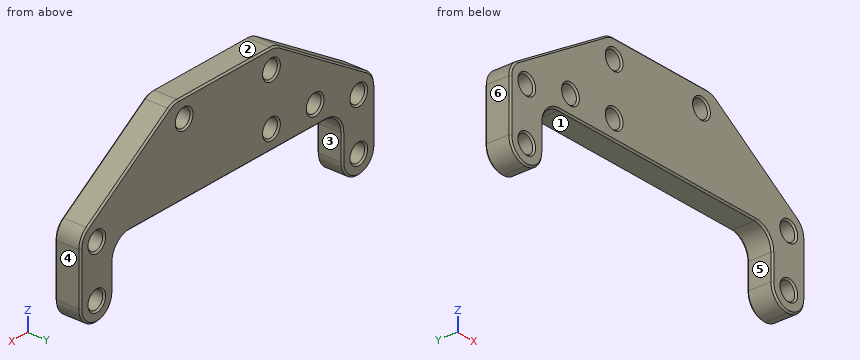
```python
from build123d import *

# Parameters (mm, degrees)
SKETCH1_R           = 2.1828125
BOSS_EXTRUDE1_DEPTH = 3.175
FILLET1_R           = 4.7625
CHAMFER1_SIZE       = 0.396875


with BuildPart() as part:
    # Sketch1 → Boss-Extrude1 (new, symmetric)
    with BuildSketch(Plane(origin=(0, 0, 0), x_dir=(1, 0, 0), z_dir=(0, 1, 0))):
        Polygon((-33.3375, 7.9375), (-33.3375, 23.8125), (-42.8625, 23.8125), (-42.8625, 3.710395607), (-14.065867028, -14.2875), (15.876245853, -14.2875), (42.8625, 3.710395607), (42.8625, 23.8125), (33.3375, 23.8125), (33.3375, 7.9375), align=None)
        with Locations(Location((-38.1, 6.35, 0), (0, 0, 270))):
            Circle(SKETCH1_R, mode=Mode.SUBTRACT)
        with Locations(Location((-38.1, 19.05, 0), (0, 0, 270))):
            Circle(SKETCH1_R, mode=Mode.SUBTRACT)
        with Locations(Location((38.1, 19.05, 0), (0, 0, 270))):
            Circle(SKETCH1_R, mode=Mode.SUBTRACT)
        with Locations(Location((38.1, 6.35, 0), (0, 0, 270))):
            Circle(SKETCH1_R, mode=Mode.SUBTRACT)
        with Locations(Location((-25.4, 3.175, 0), (0, 0, 270))):
            Circle(SKETCH1_R, mode=Mode.SUBTRACT)
        with Locations(Location((-12.7, 3.175, 0), (0, 0, 270))):
            Circle(SKETCH1_R, mode=Mode.SUBTRACT)
        with Locations(Location((-12.7, -9.525, 0), (0, 0, 270))):
            Circle(SKETCH1_R, mode=Mode.SUBTRACT)
        with Locations(Location((12.7, -9.525, 0), (0, 0, 270))):
            Circle(SKETCH1_R, mode=Mode.SUBTRACT)
    extrude(amount=BOSS_EXTRUDE1_DEPTH, both=True)

    # Fillet1
    fillet1_edges = [part.edges().sort_by_distance(p)[0] for p in [
        (42.8625, 0, -3.710395607),
        (15.876245853, 0, 14.2875),
        (-14.065867028, 0, 14.2875),
        (-42.8625, 0, -3.710395607),
        (-33.3375, 0, -23.8125),
        (-42.8625, 0, -23.8125),
        (42.8625, 0, -23.8125),
        (33.3375, 0, -23.8125),
        (33.3375, 0, -7.9375),
        (-33.3375, 0, -7.9375),
    ]]
    fillet(fillet1_edges, radius=FILLET1_R - 0.0001)  # a hair under: the kernel refuses the full size

    # Chamfer1
    chamfer1_edges = [part.edges().sort_by_distance(p)[0] for p in [
        (-38.1, -3.175, -8.5328125),
        (-38.1, 3.175, -8.5328125),
        (-38.1, -3.175, -21.2328125),
        (-38.1, 3.175, -21.2328125),
        (38.1, -3.175, -21.2328125),
        (38.1, 3.175, -21.2328125),
        (38.1, -3.175, -8.5328125),
        (38.1, 3.175, -8.5328125),
        (-12.7, -3.175, -5.3578125),
        (-12.7, 3.175, -5.3578125),
        (-25.4, -3.175, -5.3578125),
        (-25.4, 3.175, -5.3578125),
        (12.7, -3.175, 7.3421875),
        (12.7, 3.175, 7.3421875),
        (-12.7, -3.175, 7.3421875),
        (-12.7, 3.175, 7.3421875),
        (42.8625, -3.175, -12.654350033),
        (42.8625, 3.175, -12.654350033),
        (28.909389934, -3.175, 5.595327855),
        (0.866903869, -3.175, 14.2875),
        (-27.924131292, -3.175, 5.626084835),
        (-42.8625, -3.175, -12.700022288),
        (-33.3375, -3.175, -15.875),
        (0, -3.175, -7.9375),
        (33.3375, -3.175, -15.875),
        (34.732374665, -3.175, -22.417625335),
        (41.467625335, -3.175, -22.417625335),
        (-41.467625335, -3.175, -22.417625335),
        (-34.732374665, -3.175, -22.417625335),
        (-42.265497353, -3.175, -4.041282917),
        (-14.01293908, -3.175, 14.102951029),
        (15.814317137, -3.175, 14.083030095),
        (42.299190555, -3.175, -4.011804065),
        (28.909389934, 3.175, 5.595327855),
        (33.3375, 3.175, -15.875),
        (0, 3.175, -7.9375),
        (-33.3375, 3.175, -15.875),
        (-42.8625, 3.175, -12.700022288),
        (-27.924131292, 3.175, 5.626084835),
        (0.866903869, 3.175, 14.2875),
        (34.732374665, 3.175, -22.417625335),
        (41.467625335, 3.175, -22.417625335),
        (-41.467625335, 3.175, -22.417625335),
        (-34.732374665, 3.175, -22.417625335),
        (-42.265497353, 3.175, -4.041282917),
        (-14.01293908, 3.175, 14.102951029),
        (15.814317137, 3.175, 14.083030095),
        (42.299190555, 3.175, -4.011804065),
        (31.942625335, -3.175, -9.332374665),
        (31.942625335, 3.175, -9.332374665),
        (-31.942625335, -3.175, -9.332374665),
        (-31.942625335, 3.175, -9.332374665),
    ]]
    chamfer(chamfer1_edges, length=CHAMFER1_SIZE)


solid = part.part
```
Check sheet for the modelled part. Datum: model origin and axes. Units: mm. Face numbers are marked on the shaded views. A direction names the side the tool comes from. Coordinates: 2 decimals unless noted, no trailing zeros. Order: outer loops, then holes, each group sorted by start corner. A loop starts at its lowest first (then second) coordinate and runs counter-clockwise, first axis right, second up. Notation, with made-up numbers: M 79,-12.5 L 126,-12.5 A16 ccw 126,-0.5 Z; hole C -19.5,-6 d7. An arc over 180 degrees is marked long. One line per question, with ' | ' between items. Start each with the question number.
Item 1: Gauge pin test, flat ends, axial feed: P1, Ø4, axis at x = 38.1, z = -19.05, coming from the +Y side; P2, Ø2, axis at y = -1.5, z = -0.5, coming from the +X side; P3, Ø2, axis at x = 19, y = -2, coming from the +Z side; P4, Ø5, axis at x = -38.1, z = -6.35, coming from the +Y side. Record the tip position at first contact, or that the pin passes through.
Item 2: Access from +Z, -Z, +X, -X, +Y, -Y to the whole of each face (thin tool, end or side, straight path). Record for the marked faces 5 and 6.
Item 3: Mould release check, pull along X, two halves, no side actions. Record for the marked faces 1, 2, 3 and 4: pulls with the +X half, pulls with the -X half, needs draft (parallel to the pull), parting line crosses it, or undercut.
Item 4: Sectioned sample at A-A on y = 0.25. Count the separate pieces of the cut face and the enclosed holes in it, and give its area (3 significant figures).
Item 5: Sectioned sample at B-B on x = 12.7. Record the cut outline in (y, z) (1 decimal).
Item 6: Sectioned sample at C-C on z = 3. Record the cut outline in (x, y) (3 decimals), and give its area (3 significant figures).
Item 7: Material ranges on line 1 (X direction, y = 0.3, z = -19.05); line 2 (X direction, y = 1.4, z = -6.35); line 3 (X direction, y = -1.5, z = 11.5), recorded low to high.
Answer below:
1) P1: passes through | P2: stops at x = 39.55 | P3: stops at z = 12.87 | P4: stops at y = 3.1
2) face 5: -Z, +Y, -Y | face 6: +Z, -Z, -X, +Y, -Y
3) face 1: undercut | face 2: needs draft | face 3: undercut | face 4: pulls with the +X half
4) separate pieces: 1 | enclosed holes: 8 | area: 1,570 mm^2
5) outline: M -3.2,-7.5 L -2.8,-7.9 L 2.8,-7.9 L 3.2,-7.5 L 3.2,6.9 L 2.8,7.3 L -2.8,7.3 L -3.2,6.9 Z; M -3.2,12.1 L -2.8,11.7 L 2.8,11.7 L 3.2,12.1 L 3.2,13.9 L 2.8,14.3 L -2.8,14.3 L -3.2,13.9 Z
6) outline: M -32.126,-2.778 L -31.377,-3.175 L 32.086,-3.175 L 32.801,-2.778 L 32.801,2.778 L 32.086,3.175 L -31.377,3.175 L -32.126,2.778 Z | area: 412 mm^2
7) line 1: x = -42.86 to -40.28, -35.92 to -33.34, 33.34 to 35.92, 40.28 to 42.86 | line 2: x = -42.86 to -40.28, -35.92 to 35.92, 40.28 to 42.86 | line 3: x = -18.53 to -13.63, -11.77 to 11.77, 13.63 to 20.06
